Input: part model. Units: mm. Frame: model coordinates. A direction names the side the tool comes from. Round coordinates to 2 decimals unless told otherwise and drop trailing zeros. Order: outer loops, then holes, each group sorted by start corner. A loop starts at its lowest first (then second) coordinate and runs counter-clockwise, first axis right, second up. Notation, with made-up numbers: (18, -11) -> (53, -11) arc R10 cw to (53, 8) -> close; hole circle Ø7 at (13.25, 61). An arc over 180 degrees is marked (long way). Use a Markdown table: item, result.
from build123d import *

# Parameters (mm, degrees)
SKETCH_1_R      = 16
EXTRUDE_1_DEPTH = 3.5
SKETCH_2_W      = 50
SKETCH_2_H      = 20
SKETCH_2_R      = 1.5
EXTRUDE_2_DEPTH = 3
FILLET_1_R      = 2
FILLET_2_R      = 2
CHAMFER_1_SIZE  = 0.5


with BuildPart() as part:
    # 草图1 → 凸台-拉伸1 (new, symmetric)
    with BuildSketch(Plane.XY):
        with BuildLine():
            Line((17, 3), (14.406055462, 10.126804045))
            ThreePointArc((14.406055462, 10.126804045), (0, 44), (-14.406055462, 10.126804045))
            Line((-14.406055462, 10.126804045), (-17, 3))
            Line((-17, 3), (-25, 3))
            Line((-25, 3), (-25, 0))
            Line((-25, 0), (25, 0))
            Line((25, 0), (25, 3))
            Line((25, 3), (17, 3))
        make_face()
        with Locations((0, 24)):
            Circle(SKETCH_1_R, mode=Mode.SUBTRACT)
    extrude(amount=EXTRUDE_1_DEPTH, both=True)

    # 草图2 → 凸台-拉伸2 (add)
    with BuildSketch(Plane.XZ):
        Rectangle(SKETCH_2_W, SKETCH_2_H)
        with Locations(Location((-22, -7, 0), (0, 0, 270))):
            Circle(SKETCH_2_R, mode=Mode.SUBTRACT)
        with Locations(Location((22, -7, 0), (0, 0, 270))):
            Circle(SKETCH_2_R, mode=Mode.SUBTRACT)
        with Locations(Location((22, 7, 0), (0, 0, 270))):
            Circle(SKETCH_2_R, mode=Mode.SUBTRACT)
        with Locations(Location((-22, 7, 0), (0, 0, 270))):
            Circle(SKETCH_2_R, mode=Mode.SUBTRACT)
    extrude(amount=-EXTRUDE_2_DEPTH)

    # 圆角1
    fillet_1_edges = [part.edges().sort_by_distance(p)[0] for p in [
        (14.406055462, 10.126804045, 0),
        (17, 3, 0),
        (-17, 3, 0),
        (-14.406055462, 10.126804045, 0),
    ]]
    fillet(fillet_1_edges, radius=FILLET_1_R)

    # 圆角2
    fillet_2_edges = [part.edges().sort_by_distance(p)[0] for p in [
        (-25, 1.5, 10),
        (25, 1.5, 10),
        (-25, 1.5, -10),
        (25, 1.5, -10),
    ]]
    fillet(fillet_2_edges, radius=FILLET_2_R)

    # 倒角1
    chamfer_1_edges = [part.edges().sort_by_distance(p)[0] for p in [
        (-16, 24, -3.5),
        (-16, 24, 3.5),
    ]]
    chamfer(chamfer_1_edges, length=CHAMFER_1_SIZE)


solid = part.part
1) Ray query, probe 1 along X at (y, z) = (1, 7); probe 2 along Y at (x, z) = (-19, -6); probe 3 along Y at (x, z) = (9, 0). Return the intervals inside material, ascending.
Answer key:
| item | result |
|---|---|
| probe 1 | x = -25 to -23.5, -20.5 to 20.5, 23.5 to 25 |
| probe 2 | y = 0 to 3 |
| probe 3 | y = 0 to 10.77, 37.23 to 41.86 |
2) Cut plane D-D on x = 19. Return loops of the section in (y, z) (3 decimals).
Answer key:
| item | result |
|---|---|
| outline | (0, -10) -> (3, -10) -> (3, 10) -> (0, 10) -> close; (17.755, -3.5) -> (30.245, -3.5) -> (30.245, 3.5) -> (17.755, 3.5) -> close |
3) Cut plane B-B on x = -22. Return loops of the section in (y, z), and give its area (3 significant figures).
Answer key:
| item | result |
|---|---|
| outline | (0, -10) -> (3, -10) -> (3, -8.5) -> (0, -8.5) -> close; (0, -5.5) -> (3, -5.5) -> (3, 5.5) -> (0, 5.5) -> close; (0, 8.5) -> (3, 8.5) -> (3, 10) -> (0, 10) -> close |
| area | 42.0 mm^2 |
4) Cut plane A-A on z = -7. Return loops of the section in (x, y), and give its area (3 significant figures).
Answer key:
| item | result |
|---|---|
| outline | (-25, 0) -> (-23.5, 0) -> (-23.5, 3) -> (-25, 3) -> close; (-20.5, 0) -> (20.5, 0) -> (20.5, 3) -> (-20.5, 3) -> close; (23.5, 0) -> (25, 0) -> (25, 3) -> (23.5, 3) -> close |
| area | 132 mm^2 |
5) Set-up query: faces 4 (the face through (-9, 9.9, 3.5)), 5 (the face through (-17.27, 3.35, 0.05)), 6 (the face through (17.27, 3.35, -0.05)). Return all of +Z, -Z, +X, -X, +Y, -Y with unobstructed straight access to the full face (end or side cutting, diameter ignored); none if empty.
Answer key:
| item | result |
|---|---|
| face 4 | +Z, +X, -X, +Y |
| face 5 | +Z, -Z, -X |
| face 6 | +Z, -Z, +X |
6) Contact query for flat-ended pins moving along their axis: P1, Ø8, axis at y = 15.5, z = -8, coming from the -X side; P2, Ø6, axis at y = 30.5, z = 4, coming from the +X side; P3, Ø5, axis at x = -9, y = 38, coming from the -Z side; P4, Ø5, axis at x = 5.5, z = -8, coming from the +Y side. Output: stop coordinate, or through.
Answer key:
| item | result |
|---|---|
| P1 | passes through |
| P2 | stops at x = 19.68 |
| P3 | stops at z = -3.5 |
| P4 | stops at y = 3 |
7) Draft query along Z for faces 1 (the face through (-15.658, 6.687, 0.049)), 2 (the face through (24.43, 1.52, -9.4)), 3 (the face through (23.01, 1.48, -5.89)). Return one class per face: released by +Z, released by -Z, zero draft, split by the parting line, or undercut.
Answer key:
| item | result |
|---|---|
| face 1 | zero draft |
| face 2 | released by -Z |
| face 3 | undercut |
8) Cut plane C-C on z = -1.75. Return loops of the section in (x, y), and give its area (3 significant figures).
Answer key:
| item | result |
|---|---|
| outline | (-25, 0) -> (25, 0) -> (25, 3) -> (18.4, 3) arc R2 cw to (16.52, 4.32) -> (14.82, 8.99) arc R2 cw to (15.18, 10.98) arc R20 ccw (long way) to (-15.18, 10.98) arc R2 cw to (-14.82, 8.99) -> (-16.52, 4.32) arc R2 cw to (-18.4, 3) -> (-25, 3) -> close; hole circle Ø32 at (0, 24) |
| area | 706 mm^2 |
